Can you work these out from the model? Positions are in its coordinate system, mm. Face numbers are marked on the shaded views. A direction names the side the tool comes from. Give positions to 0.01 mm unless a question says otherwise; leave off trailing zeros. Loops run counter-clockwise (first coordinate to the right, second up) from the corner with the lowest first, then second, coordinate; pieces in that order, holes last. Notation, with made-up numbers: (29, 26) - (48, 26) arc R30 ccw to (48, 64) - close; hole circle Ø11 at (28.5, -18.75). An arc over 180 degrees is marked (long way). Answer in a Markdown table with one row per item.
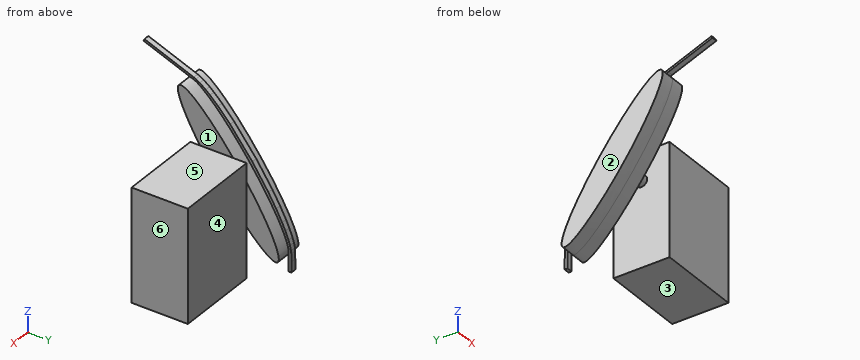
from build123d import *

# Parameters (mm, degrees)
SKETCH_1_W      = 30
SKETCH_1_H      = 20
EXTRUDE_1_DEPTH = 40
SKETCH_2_R      = 2
EXTRUDE_2_DEPTH = 5
SKETCH_3_RX     = 30
SKETCH_3_RY     = 5
EXTRUDE_3_DEPTH = 5
EXTRUDE_4_DEPTH = 2
EXTRUDE_5_DEPTH = 5


# Read off the part's stored shape, not the designer's step: the extrude step
with BuildPart() as part:
    # Sketch 1 → Extrude 1 (new body)
    with BuildSketch(Plane.XY):
        with Locations((15, 10)):
            Rectangle(SKETCH_1_W, SKETCH_1_H)
    extrude(amount=EXTRUDE_1_DEPTH)

    # Sketch 2 → Extrude 2 (add)
    with BuildSketch(Plane.ZY):
        with Locations(Location((30, 10, 0), (0, 0, 180))):
            Circle(SKETCH_2_R)
    extrude(amount=EXTRUDE_2_DEPTH)

    # Sketch 3 → Extrude 3 (add)
    with BuildSketch(Plane.ZY.offset(5)):
        with Locations(Location((30, 10), (0, 0, 144.330167024))):
            Ellipse(SKETCH_3_RX, SKETCH_3_RY)
    extrude(amount=EXTRUDE_3_DEPTH)



with BuildPart() as body_2:
    # Sketch 4 → Extrude 4 (new body)
    with BuildSketch(Plane.ZY.offset(10)):
        with BuildLine():
            add(Edge.make_bspline(
                [(6.506952715, 28.909855834), (5.513332822, 28.917697958), (4.992779523, 28.561751889)],
                knots=[6.015569415, 6.015569415, 6.015569415, 6.212983263, 6.212983263, 6.212983263], degree=2, weights=[1, 0.995132426, 1]))
            Line((4.992779523, 28.561751889), (7.137480457, 27.953085866))
            add(Edge.make_bspline(
                [(8.41739908, 27.759268462), (7.691843708, 27.924954947), (7.137480457, 27.953085866)],
                knots=[5.905821209, 5.905821209, 5.905821209, 6.029787374, 6.029787374, 6.029787374], degree=2, weights=[1, 0.998079664, 1]))
            add(Edge.make_bspline(
                [(9.931154304, 27.32571063), (9.102712315, 27.602771598), (8.41739908, 27.759268462)],
                knots=[5.788714528, 5.788714528, 5.788714528, 5.905821209, 5.905821209, 5.905821209], degree=2, weights=[1, 0.998286243, 1]))
            add(Edge.make_bspline(
                [(12.213928034, 26.448131332), (10.970222869, 26.978208516), (9.931154304, 27.32571063)],
                knots=[5.641930178, 5.641930178, 5.641930178, 5.788714528, 5.788714528, 5.788714528], degree=2, weights=[1, 0.997308003, 1]))
            add(Edge.make_bspline(
                [(17.511716763, 23.85284507), (14.569327703, 25.444240976), (12.213928034, 26.448131332)],
                knots=[5.365220638, 5.365220638, 5.365220638, 5.641930178, 5.641930178, 5.641930178], degree=2, weights=[1, 0.990444236, 1]))
            add(Edge.make_bspline(
                [(21.663153618, 21.483483589), (19.49565109, 22.779830964), (17.511716763, 23.85284507)],
                knots=[5.17799572, 5.17799572, 5.17799572, 5.365220638, 5.365220638, 5.365220638], degree=2, weights=[1, 0.995621553, 1]))
            add(Edge.make_bspline(
                [(28.161833123, 17.358582765), (24.817516303, 19.596911494), (21.663153618, 21.483483589)],
                knots=[4.906410628, 4.906410628, 4.906410628, 5.17799572, 5.17799572, 5.17799572], degree=2, weights=[1, 0.990794351, 1]))
            add(Edge.make_bspline(
                [(31.719121271, 14.913354973), (29.940162996, 16.168358555), (28.161833123, 17.358582765)],
                knots=[4.761356742, 4.761356742, 4.761356742, 4.906410628, 4.906410628, 4.906410628], degree=2, weights=[1, 0.997371074, 1]))
            add(Edge.make_bspline(
                [(37.988291289, 10.282541681), (34.937566868, 12.642834742), (31.719121271, 14.913354973)],
                knots=[4.4999664, 4.4999664, 4.4999664, 4.761356742, 4.761356742, 4.761356742], degree=2, weights=[1, 0.991471536, 1]))
            add(Edge.make_bspline(
                [(44.627089911, 4.844191407), (41.578227004, 7.505070109), (37.988291289, 10.282541681)],
                knots=[4.193044565, 4.193044565, 4.193044565, 4.4999664, 4.4999664, 4.4999664], degree=2, weights=[1, 0.988247964, 1]))
            add(Edge.make_bspline(
                [(50.343902664, -0.577200355), (47.99639472, 1.903648758), (44.627089911, 4.844191407)],
                knots=[3.854449116, 3.854449116, 3.854449116, 4.193044565, 4.193044565, 4.193044565], degree=2, weights=[1, 0.985703337, 1]))
            add(Edge.make_bspline(
                [(52.4832091, -3.016334631), (51.589789327, -1.893854823), (50.343902664, -0.577200355)],
                knots=[3.673505786, 3.673505786, 3.673505786, 3.854449116, 3.854449116, 3.854449116], degree=2, weights=[1, 0.99591023, 1]))
            add(Edge.make_bspline(
                [(53.450493398, -4.328804293), (53.040359197, -3.716330033), (52.4832091, -3.016334631)],
                knots=[3.56047839, 3.56047839, 3.56047839, 3.673505786, 3.673505786, 3.673505786], degree=2, weights=[1, 0.998403526, 1]))
            add(Edge.make_bspline(
                [(54.25730413, -5.755095942), (53.982230556, -5.122874432), (53.450493398, -4.328804293)],
                knots=[3.414044896, 3.414044896, 3.414044896, 3.56047839, 3.56047839, 3.56047839], degree=2, weights=[1, 0.997320851, 1]))
            add(Edge.make_bspline(
                [(54.515784231, -6.566048985), (54.452837221, -6.2045038), (54.25730413, -5.755095942)],
                knots=[3.309862159, 3.309862159, 3.309862159, 3.414044896, 3.414044896, 3.414044896], degree=2, weights=[1, 0.998643551, 1]))
            Line((54.515784231, -6.566048985), (55.035975621, -7.912515095))
            add(Edge.make_bspline(
                [(55.035975621, -7.912515095), (55.571319453, -7.205458838), (55.0082883, -5.755095942)],
                knots=[3.136655758, 3.136655758, 3.136655758, 3.430060288, 3.430060288, 3.430060288], degree=2, weights=[1, 0.989258508, 1]))
            Line((55.0082883, -5.755095942), (54.668462814, -5.006548181))
            Line((54.668462814, -5.006548181), (53.860777814, -3.651060405))
            Line((53.860777814, -3.651060405), (52.255398503, -1.516776462))
            Line((52.255398503, -1.516776462), (50.940415781, 0))
            Line((50.940415781, 0), (48.186919212, 2.84562684))
            Line((48.186919212, 2.84562684), (43.454466091, 7.163503062))
            Line((43.454466091, 7.163503062), (33.368126059, 15.062192859))
            Line((33.368126059, 15.062192859), (24.869605616, 20.749286032))
            Line((24.869605616, 20.749286032), (20.147321799, 23.537005238))
            Line((20.147321799, 23.537005238), (16.169043828, 25.636582623))
            Line((16.169043828, 25.636582623), (13.69703985, 26.794407183))
            Line((13.69703985, 26.794407183), (10.928759246, 27.90628218))
            Line((10.928759246, 27.90628218), (9.248929013, 28.444330815))
            Line((9.248929013, 28.444330815), (7.585869147, 28.814585944))
            Line((7.585869147, 28.814585944), (6.506952715, 28.909855834))
        make_face()
        with BuildLine():
            Line((3.687796669, 28.932105961), (4.992779523, 28.561751889))
            add(Edge.make_bspline(
                [(6.506952715, 28.909855834), (5.513332822, 28.917697958), (4.992779523, 28.561751889)],
                knots=[6.015569415, 6.015569415, 6.015569415, 6.212983263, 6.212983263, 6.212983263], degree=2, weights=[1, 0.995132426, 1]))
            Line((6.506952715, 28.909855834), (3.687796669, 28.932105961))
        make_face()
        with BuildLine():
            Line((0, 28.264369192), (4.685334353, 28.264369192))
            add(Edge.make_bspline(
                [(4.992779523, 28.561751889), (4.808192105, 28.435533949), (4.685334353, 28.264369192)],
                knots=[6.212983263, 6.212983263, 6.212983263, 6.283185307, 6.283185307, 6.283185307], degree=2, weights=[1, 0.999384022, 1]))
            Line((4.992779523, 28.561751889), (3.687796669, 28.932105961))
            Line((3.687796669, 28.932105961), (0, 28.961211815))
            Line((0, 28.961211815), (0, 28.264369192))
        make_face()
        with BuildLine():
            add(Edge.make_bspline(
                [(4.685334353, 28.264369192), (4.57062955, 28.10456308), (4.510252037, 27.90628218)],
                knots=[0, 0, 0, 0.065546828, 0.065546828, 0.065546828], degree=2, weights=[1, 0.999463, 1]))
            Line((4.685334353, 28.264369192), (0, 28.264369192))
            Line((0, 28.264369192), (0, 27.90628218))
            Line((0, 27.90628218), (4.510252037, 27.90628218))
        make_face()
        with BuildLine():
            add(Edge.make_bspline(
                [(4.992779523, 28.561751889), (4.808192105, 28.435533949), (4.685334353, 28.264369192)],
                knots=[6.212983263, 6.212983263, 6.212983263, 6.283185307, 6.283185307, 6.283185307], degree=2, weights=[1, 0.999384022, 1]))
            add(Edge.make_bspline(
                [(4.685334353, 28.264369192), (4.57062955, 28.10456308), (4.510252037, 27.90628218)],
                knots=[0, 0, 0, 0.065546828, 0.065546828, 0.065546828], degree=2, weights=[1, 0.999463, 1]))
            Line((4.510252037, 27.90628218), (6.34848035, 27.90628218))
            add(Edge.make_bspline(
                [(7.137480457, 27.953085866), (6.682690118, 27.976164001), (6.34848035, 27.90628218)],
                knots=[6.029787374, 6.029787374, 6.029787374, 6.131529727, 6.131529727, 6.131529727], degree=2, weights=[1, 0.998706341, 1]))
            Line((7.137480457, 27.953085866), (4.992779523, 28.561751889))
        make_face()
        with BuildLine():
            add(Edge.make_bspline(
                [(55.035975621, -7.912515095), (55.571319453, -7.205458838), (55.0082883, -5.755095942)],
                knots=[3.136655758, 3.136655758, 3.136655758, 3.430060288, 3.430060288, 3.430060288], degree=2, weights=[1, 0.989258508, 1]))
            Line((55.035975621, -7.912515095), (61.090316434, -23.583602479))
            Line((61.090316434, -23.583602479), (61.819897807, -23.301737273))
            Line((61.819897807, -23.301737273), (55.0082883, -5.755095942))
        make_face()
    extrude(amount=EXTRUDE_4_DEPTH)


with BuildPart() as part_1:
    add(part.part)

    add(body_2.part)  # Extrude 5 merges body 2
    # Extrude 5 outline → Extrude 5 (add)
    with BuildSketch(Plane.ZY.offset(10)):
        with BuildLine():
            add(Edge.make_bspline(
                [(54.371719706, -7.493406717), (54.465505659, -7.362744634), (54.529944837, -7.206425025), (54.561913477, -7.022620585), (54.558192199, -6.809625231), (54.202681657, -4.767699434), (51.727605158, -1.240686466), (46.200440793, 4.025468627), (39.039651813, 9.679286683), (26.386377317, 18.734970385), (18.758776419, 23.664893419), (12.075170793, 27.137730816), (8.050806871, 28.262231314), (4.642942369, 27.549661544), (4.877580773, 25.652182817), (7.730736464, 22.205445776), (11.438087078, 18.596318521), (22.095709136, 9.277375664), (34.757298876, -0.521475217), (47.784810652, -8.095593664), (53.361737398, -8.90050861), (54.371719706, -7.493406717)],
                knots=[0, 0, 0, 0, 0, 0, 0.194483448, 0.194483448, 0.194483448, 0.194483448, 1.630375604, 1.630375604, 1.630375604, 1.630375604, 3.066267761, 3.066267761, 3.066267761, 3.066267761, 4.504868745, 4.504868745, 4.504868745, 4.504868745, 7.04748776, 7.04748776, 7.04748776, 7.04748776, 7.04748776, 7.04748776], degree=5, weights=[1, 1, 1.000007219, 1.000006403, 1, 1, 0.977216815, 0.977216815, 1, 1, 0.977216815, 0.977216815, 1, 1, 0.990702131, 0.997630061, 1, 1, 0.9, 0.9, 1, 1]))
        make_face()
    extrude(amount=EXTRUDE_5_DEPTH)


solid = part_1.part
Q1. On a 3-axis mill with a long thin cutter (end or side, diameter ignored), from which of +Z, -Z, +X, -X, +Y, -Y can I reach the whole of each face in a straight line? I mean the marked faces 4, 5 and 6. Say none if no direction works.
Checked values:
| item | result |
|---|---|
| face 4 | +Z, -Z, +X, +Y |
| face 5 | +Z, +X, +Y, -Y |
| face 6 | +Z, -Z, +X, +Y, -Y |
Q2. If we mould it in two halves opening along X, with no side actions, what happens to the marked faces 1, 2 and 3? For each: released by +X, released by -X, zero draft, split by the parting line, or undercut.
Checked values:
| item | result |
|---|---|
| face 1 | undercut |
| face 2 | released by -X |
| face 3 | zero draft |
Q3. Imagine slicing it at B-B, the plane x = 17. Write out the boundary of the cut face in (y, z), and give its area (3 significant figures).
Checked values:
| item | result |
|---|---|
| outline | (0, 0) - (20, 0) - (20, 40) - (0, 40) - close |
| area | 800 mm² |
Q4. For pin 1 (6 mm diameter, centred on x = 11.5, y = 12, fed in from +Z); pin 2 (3 mm diameter, centred on x = 21, z = 16.5, fed in from -Y); pin 3 (6 mm diameter, centred on y = 6, z = 21.5, fed in from -X), each with a flat end and sliding along its axis, tell me the tip position at first contact or that it passes through.
Checked values:
| item | result |
|---|---|
| pin 1 | stops at z = 40 |
| pin 2 | stops at y = 0 |
| pin 3 | stops at x = 0 |
Q5. If I drill on line 1 (Z direction, x = 7, y = 6); line 2 (Y direction, x = 26, z = 31.5); line 3 (Z direction, x = -3, y = 10), over which ranges is the centre line in solid material (lowest first)? Write a range as [from, to].
Checked values:
| item | result |
|---|---|
| line 1 | z = [0, 40] |
| line 2 | y = [0, 20] |
| line 3 | z = [28, 32] |
Q6. Imagine slicing it at A-A, the plane y = -14.5. Write out the boundary of the cut face in (x, z).
Checked values:
| item | result |
|---|---|
| outline | (-12, 57.58) - (-10, 57.58) - (-10, 58.4) - (-12, 58.4) - close |
